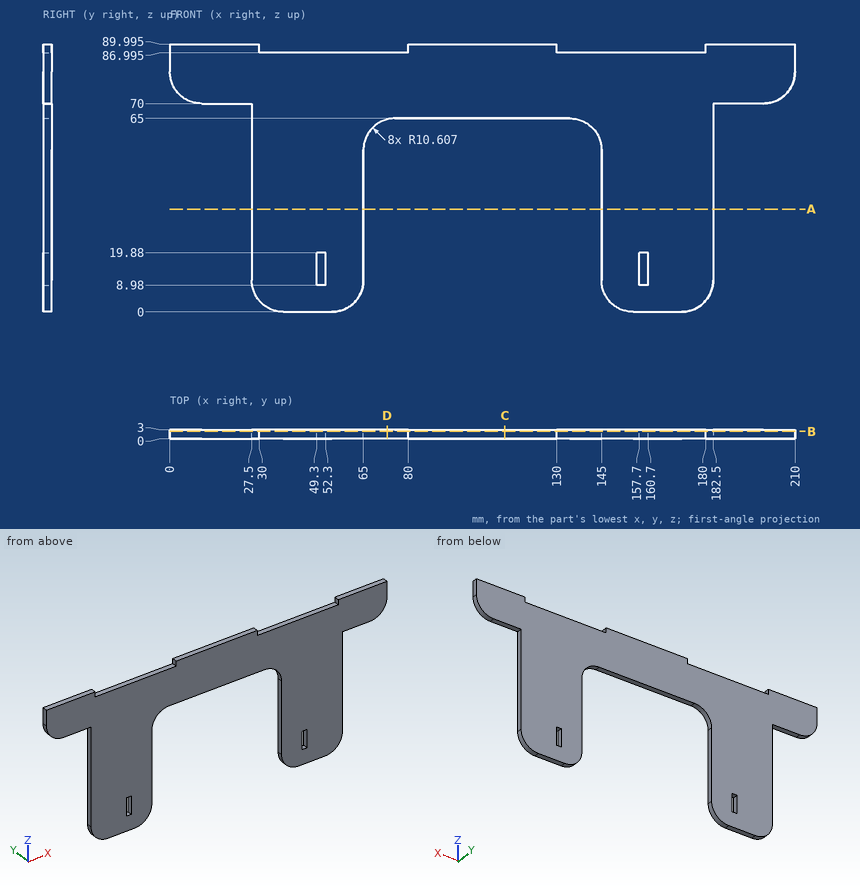
Verification items for this drawing (mm, ordinates from the low corner). Coordinates: 2 decimals unless noted, no trailing zeros. Loops run counter-clockwise (first coordinate to the right, second up) from the corner with the lowest first, then second, coordinate; pieces in that order, holes last.
Item 1: Sectioned sample at A-A, the plane z = 34.5. Record the boundary of the cut face in (x, y).
Item 2: Sectioned sample at C-C, the plane x = 112.5. Record the boundary of the cut face in (y, z) (1 decimal).
Item 3: Sectioned sample at D-D, the plane x = 73. Record the boundary of the cut face in (y, z) (1 decimal).
Item 4: Go/stop test with flat-tipped pins: pin 1 Ø1.5 at (x, y) = (97.5, 1.5) entering from -Z; pin 2 Ø3 at (x, z) = (151, 23.5) entering from -Y; pin 3 Ø1.5 at (x, y) = (24, 1) entering from -Z; pin 4 Ø1.5 at (x, y) = (51, 2) entering from +Z (1 decimal). Record where each tip stops, or that it passes through.
Item 5: Sectioned sample at B-B, the plane y = 2.5. Count the separate pieces of the cut face and the enclosed holes in it, then the cut area to 3 significant figures.
Item 6: Thickness scan on line 1 (X direction, y = 1.4, z = 15.5); line 2 (X direction, y = 2.8, z = 21); line 3 (Z direction, x = 103, y = 0.25) (1 decimal). Record the ranges inside material, lowest first.
Check result:
1. outline: (27.5, 0) - (65, 0) - (65, 3) - (27.5, 3) - close; (145, 0) - (182.5, 0) - (182.5, 3) - (145, 3) - close
2. outline: (0, 65) - (3, 65) - (3, 90) - (0, 90) - close
3. outline: (0, 64.7) - (3, 64.7) - (3, 87) - (0, 87) - close
4. pin 1: stops at z = 65
4. pin 2: stops at y = 0
4. pin 3: stops at z = 70
4. pin 4: stops at z = 87
5. separate pieces: 1
5. enclosed holes: 2
5. area: 9,390 mm2
6. line 1: x = 27.5 to 49.3, 52.3 to 65, 145 to 157.7, 160.7 to 182.5
6. line 2: x = 27.5 to 65, 145 to 182.5
6. line 3: z = 65 to 90
